Input: part model. Units: mm. Frame: model coordinates. Round coordinates to 2 decimals unless told otherwise and drop trailing zeros. Order: outer loops, then holes, each group sorted by start corner. A loop starts at its lowest first (then second) coordinate and runs counter-clockwise, first axis right, second up.
Item 1: Line query: L1, parallel to X at y = 0.9, z = -194.5; L2, parallel to Z at x = 357, y = 2.05; L3, parallel to X at y = 1.8, z = -65.5. Output: solid intervals per line, ascending.
Item 2: Cut plane A-A on x = 118. Output: boundary loops of the cut face in (y, z).
Item 3: Cut plane B-B on y = 0.95. Give the number of separate pieces and of enclosed holes in the cut face, then the cut area to 3 significant figures.
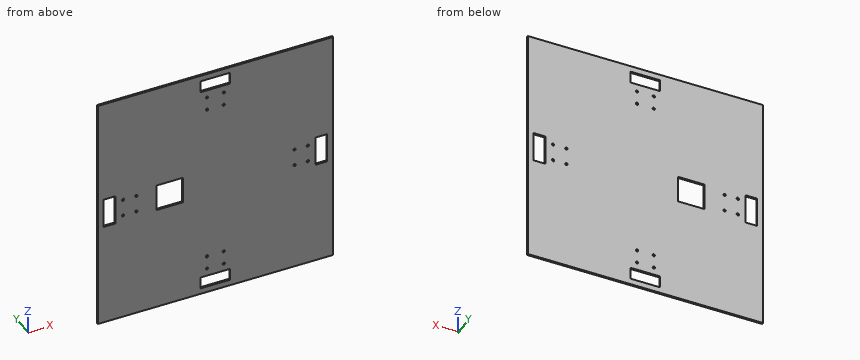
```python
from build123d import *

# Parameters (mm, degrees)
SKETCH1_W      = 400
SKETCH1_H      = 400
SKETCH1_R      = 2
SKETCH1_W_2    = 20
SKETCH1_H_2    = 50
SKETCH1_W_3    = 50
SKETCH1_H_3    = 20
SKETCH1_W_4    = 45
SKETCH1_H_4    = 45
EXTRUDE1_DEPTH = 3


with BuildPart() as part:
    # Sketch1 → Extrude1 (new body)
    with BuildSketch(Plane(origin=(0, 0, 0), x_dir=(1, 0, 0), z_dir=(0, 1, 0))):
        with Locations((200, 200)):
            Rectangle(SKETCH1_W, SKETCH1_H)
        with Locations(Location((185.75, 43, 0), (0, 0, 270))):
            Circle(SKETCH1_R, mode=Mode.SUBTRACT)
        with Locations(Location((185.75, 65.5, 0), (0, 0, 270))):
            Circle(SKETCH1_R, mode=Mode.SUBTRACT)
        with Locations(Location((214.25, 65.5, 0), (0, 0, 90))):
            Circle(SKETCH1_R, mode=Mode.SUBTRACT)
        with Locations(Location((214.25, 43, 0), (0, 0, 90))):
            Circle(SKETCH1_R, mode=Mode.SUBTRACT)
        with Locations(Location((43, 214.25, 0), (0, 0, 270))):
            Circle(SKETCH1_R, mode=Mode.SUBTRACT)
        with Locations(Location((65.5, 214.25, 0), (0, 0, 270))):
            Circle(SKETCH1_R, mode=Mode.SUBTRACT)
        with Locations(Location((65.5, 185.75, 0), (0, 0, 90))):
            Circle(SKETCH1_R, mode=Mode.SUBTRACT)
        with Locations(Location((43, 185.75, 0), (0, 0, 90))):
            Circle(SKETCH1_R, mode=Mode.SUBTRACT)
        with Locations(Location((214.25, 357, 0), (0, 0, 270))):
            Circle(SKETCH1_R, mode=Mode.SUBTRACT)
        with Locations(Location((214.25, 334.5, 0), (0, 0, 270))):
            Circle(SKETCH1_R, mode=Mode.SUBTRACT)
        with Locations(Location((185.75, 334.5, 0), (0, 0, 90))):
            Circle(SKETCH1_R, mode=Mode.SUBTRACT)
        with Locations(Location((185.75, 357, 0), (0, 0, 90))):
            Circle(SKETCH1_R, mode=Mode.SUBTRACT)
        with Locations(Location((357, 185.75, 0), (0, 0, 270))):
            Circle(SKETCH1_R, mode=Mode.SUBTRACT)
        with Locations(Location((334.5, 185.75, 0), (0, 0, 270))):
            Circle(SKETCH1_R, mode=Mode.SUBTRACT)
        with Locations(Location((334.5, 214.25, 0), (0, 0, 90))):
            Circle(SKETCH1_R, mode=Mode.SUBTRACT)
        with Locations(Location((357, 214.25, 0), (0, 0, 90))):
            Circle(SKETCH1_R, mode=Mode.SUBTRACT)
        with Locations((20, 200)):
            Rectangle(SKETCH1_W_2, SKETCH1_H_2, mode=Mode.SUBTRACT)
        with Locations((200, 20)):
            Rectangle(SKETCH1_W_3, SKETCH1_H_3, mode=Mode.SUBTRACT)
        with Locations((200, 380)):
            Rectangle(SKETCH1_W_3, SKETCH1_H_3, mode=Mode.SUBTRACT)
        with Locations((380, 200)):
            Rectangle(SKETCH1_W_2, SKETCH1_H_2, mode=Mode.SUBTRACT)
        with Locations((122.5, 200)):
            Rectangle(SKETCH1_W_4, SKETCH1_H_4, mode=Mode.SUBTRACT)
    extrude(amount=EXTRUDE1_DEPTH)


solid = part.part
```
From the geometry:
1. L1: x = 0 to 10, 30 to 100, 145 to 370, 390 to 400
1. L2: z = -400 to -216.25, -212.25 to -187.75, -183.75 to 0
1. L3: x = 0 to 183.75, 187.75 to 212.25, 216.25 to 400
2. outline: (0, -400) - (3, -400) - (3, -222.5) - (0, -222.5) - close; (0, -177.5) - (3, -177.5) - (3, 0) - (0, 0) - close
3. separate pieces: 1
3. enclosed holes: 21
3. area: 154,000 mm2
